Model file for the job. Use its own axes, mm. Give positions to 0.01 mm unless a question says otherwise; leave off trailing zeros. Order: outer loops, then holes, each group sorted by start corner. A loop starts at its lowest first (then second) coordinate and runs counter-clockwise, first axis right, second up. Notation, with made-up numbers: (-31, 67.5) - (-16, 67.5) arc R19 cw to (-16, 94.5) - close; hole circle Ø7 at (-0.5, 72). An arc over 180 degrees is marked (long way). Use CSV: the item, a comma, the result in double quotes. Start each with the question number.
(1) Band-saw the part on D-D, the plane z = 23. Give the cut face in (x, y), then the cut area to 3 significant figures.
(2) Drop flat-ended pins along their axis: pin 1 Ø10 at (x, y) = (169, 58.5) entering from +Z; pin 2 Ø12 at (x, z) = (93, 10.5) entering from -Y; pin 3 Ø5 at (y, z) = (-3.5, 10.5) entering from +X. Give the stop position or say it passes through.
(3) Pull direction Y, two halves, no side cores. Call faces 1 (the flat face through (148, 65.368, 0)), 2 (the flat face through (262, -14, 32.413)), 3 (the cylindrical face through (275.98, -10.28, 19.74)), 4 (the cylindrical face through (147.9, 35.694, 1.704)): +Y half, -Y half, draft (parallel to the pull), parting line (faces both ways), or undercut.
(4) Band-saw the part on A-A, the plane x = 29. Give the cut face in (y, z).
(5) Band-saw the part on C-C, the plane x = 268.5. Give the cut face in (y, z), then the cut area to 3 significant figures.
(6) Band-saw the part on B-B, the plane y = -8.5. Give the cut face in (x, z).
(7) Probe L1, parallel to Z at x = 172.5, y = -34.5; L2, parallel to Y at x = 53, z = 5.5; L3, parallel to Y at x = 265, z = 19. List the from-to ranges inside material, lowest first.
from build123d import *

# Parameters (mm, degrees)
F1_DEPTH = 300
F2_R     = 14.602724
F3_DEPTH = 25


with BuildPart() as f1:
    # F0 (on Right) → F1 (new body)
    with BuildSketch(Plane.YZ):
        with BuildLine():
            Line((29.858291, 7.412897), (-65.36828, 7.412897))
            Line((-65.36828, 7.412897), (-65.36828, -7.412897))
            Line((-65.36828, -7.412897), (65.36828, -7.412897))
            Line((65.36828, -7.412897), (65.36828, 7.412897))
            Line((65.36828, 7.412897), (56.092858, 7.412897))
            ThreePointArc((56.092858, 7.412897), (50.38289, 1.702929), (44.672921, 7.412897))
            Line((44.672921, 7.412897), (41.278228, 7.412897))
            ThreePointArc((41.278228, 7.412897), (35.56826, 1.702929), (29.858291, 7.412897))
        make_face()
    extrude(amount=F1_DEPTH)

    # F2 (on face) → F3 (join)
    with BuildSketch(Plane.XY.offset(7.412897)):
        with Locations((262.049705, -14.663358)):
            Circle(F2_R)
    extrude(amount=F3_DEPTH)


solid = f1.part
Answer block:
1,outline,"circle Ø29.21 at (262.05, -14.66)"
1,area,"670 mm2"
2,pin 1,"stops at z = 7.41"
2,pin 2,"stops at y = -65.37"
2,pin 3,"stops at x = 273.8"
3,face 1,"+Y half"
3,face 2,"draft"
3,face 3,"parting line"
3,face 4,"undercut"
4,outline,"(-65.37, -7.41) - (65.37, -7.41) - (65.37, 7.41) - (56.09, 7.41) arc R5.71 cw to (44.67, 7.41) - (41.28, 7.41) arc R5.71 cw to (29.86, 7.41) - (-65.37, 7.41) - close"
5,outline,"(-65.37, -7.41) - (65.37, -7.41) - (65.37, 7.41) - (56.09, 7.41) arc R5.71 cw to (44.67, 7.41) - (41.28, 7.41) arc R5.71 cw to (29.86, 7.41) - (-1.56, 7.41) - (-1.56, 32.41) - (-27.76, 32.41) - (-27.76, 7.41) - (-65.37, 7.41) - close"
5,area,"2,490 mm2"
6,outline,"(0, -7.41) - (300, -7.41) - (300, 7.41) - (275.29, 7.41) - (275.29, 32.41) - (248.81, 32.41) - (248.81, 7.41) - (0, 7.41) - close"
7,L1,"z = -7.41 to 7.41"
7,L2,"y = -65.37 to 30.19, 40.95 to 45, 55.76 to 65.37"
7,L3,"y = -28.96 to -0.36"
